Autodesk Inventor part; units mm, degrees
ref_plane "YZ Plane" through (0, 0, 0) normal (1, 0, 0) x (0, 1, 0)
ref_plane "XZ Plane" through (0, 0, 0) normal (0, 1, 0) x (-1, 0, 0)
ref_plane "XY Plane" through (0, 0, 0) normal (0, 0, 1) x (1, 0, 0)
sketch "Sketch1" plane through (0, 0, 0) normal (0, 1, 0) x (-1, 0, 0)
  circle A0 centre (0, 0) radius 10
  circle A1 centre (0, 0) radius 5
  dimension "d0" = 20
extrude "Extrusion1" add sketch "Sketch1" along normal blind 4
sketch "Sketch2" plane through (0, 4, 0) normal (0, 1, 0) x (1, 0, 0)
  circle A0 centre (0, 0) radius 10
  line L0 (-10, 0) -> (10, 0)
  line L1 (10, 0) -> (10, 50)
  line L2 (10, 50) -> (-10, 50)
  line L3 (-10, 50) -> (-10, 0)
  dimension "d3" = 50
extrude "Extrusion2" add sketch "Sketch2" against normal blind 4 contours A0 L3 L2 L1
sketch "Sketch3" plane through (0, 4, 0) normal (0, 1, 0) x (1, 0, 0)
  line L0 (-10, 50) -> (10, 50)
  circle A0 centre (0, 50) radius 10
  point P0 (0, 0)
  point P1 (-10, 50)
  dimension "d19" = 20
extrude "Extrusion3" add sketch "Sketch3" against normal blind 4 contours A0 L0 picked at (2.78, 54.5572)
sketch "Sketch5" plane through (0, 4, 0) normal (0, 1, 0) x (1, 0, 0)
  arc A0 (-10, 0) -> (10, 0) centre (0, 0) ccw
  line L0 (-10, 0) -> (-10, 50)
  arc A1 (-10, 0) -> (-10, 50) centre (-86.125, 25) ccw
  line L1 (10, 50) -> (10, 0)
  arc A2 (10, 50) -> (10, 0) centre (86.125, 25) ccw
extrude "Extrusion4" cut sketch "Sketch5" against normal blind 4
fillet "Fillet1" radius 2 1 edges at (10, 2, -50)
fillet "Fillet2" radius 2 1 edges at (-10, 2, -50)
fillet "Fillet3" radius 2 1 edges at (-10, 2, 0)
fillet "Fillet4" radius 2 1 edges at (10, 2, 0)
sketch "Sketch6" plane through (0, 4, 0) normal (0, 1, 0) x (1, 0, 0)
  arc A0 (9.9929, 50.3757) -> (-9.9929, 50.3757) centre (0, 50) ccw
  circle A1 centre (0, 50) radius 2.5
  point P0 (0, 0)
  dimension "d14" = 5
extrude "Extrusion5" cut sketch "Sketch6" against normal blind 4
fillet "Fillet5" radius 2 5 edges at (0, 4, -60) (-9.9754, 4, 0.0258) (0, 4, 10) (9.9754, 4, 0.0258) (6, 4, -25)
fillet "Fillet6" radius 2 5 edges at (0, 0, -60) (6, 0, -25) (9.9754, 0, 0.0258) (0, 0, 10) (-9.9754, 0, 0.0258)
properties part number "Arm"
Part model, mm, in its own coordinate system. Coordinates: 2 decimals unless noted, no trailing zeros. Put each result on its own line as item: value.
1. Flat gauge pin, fed straight in: pin 1 Ø8 at (x, z) = (0, -50) entering from +Y. Where does the tip first touch, or does it go through?
Final values:
pin 1: stops at y = 4
2. Probe line 1 along Z through (x, y) = (2.25, 2.3); line 2 along Z through (x, y) = (0, 1.35); line 3 along X through (y, z) = (1.1, -1.5). List the from-to ranges inside material, lowest first. Write a range as [from, to].
Final values:
line 1: z = [-59.72, -51.09], [-48.91, -4.47], [4.47, 9.72]
line 2: z = [-59.89, -52.5], [-47.5, -5], [5, 9.89]
line 3: x = [-9.3, -4.77], [4.77, 9.3]
3. Band-saw the part on A-A (x = 0). Give the number of separate pieces and of enclosed holes in the cut face, then the cut area to 3 significant figures.
Final values:
separate pieces: 3
enclosed holes: 0
area: 217 mm²
4. Two-plate mould, pull along Z, no slides. Class faces 1 (the flat face through (0, 4, -25)), 2 (the cylindrical face through (-0.54, 2.03, -47.56)), 3 (the cylindrical face through (1.08, 1.97, 4.88)): +Z half, -Z half, draft (parallel to the pull), parting line (faces both ways), or undercut.
Final values:
face 1: draft
face 2: undercut
face 3: undercut
